Could you check a few things on this model? Use its own coordinates, in mm. Face numbers are marked on the shaded views. Give positions to 0.01 mm unless a question says otherwise; leave off trailing zeros. Loops run counter-clockwise (first coordinate to the right, second up) from the corner with the lowest first, then second, coordinate; pieces in that order, holes last. Notation, with made-up numbers: (71, 85.25) -> (124, 85.25) arc R18 cw to (124, 119.25) -> close; hole circle Ø5 at (-12, 87). An arc over 180 degrees is marked (long way). Write each question's results on one line, items separated by ' | '. Start each with the question number.
Q1. If we section it at A-A, the plane x = 0: List the corners of the cut face in (y, z) for me, plus the area to 3 significant figures.
Q2. Will these pins go through, and if not, where does the flat tip stop? P1, Ø1.5, axis at y = 3.5, z = -0.5, coming from the -X side; P2, Ø1.5, axis at x = -17, y = 3, coming from the +Z side; P3, Ø3, axis at x = 14.5, z = -14, coming from the +Y side.
Q3. If we section it at C-C, the plane y = 7: List the corners of the cut face in (x, z) for me.
Q4. If we section it at B-B, the plane z = 0: List the corners of the cut face in (x, y) for me.
Q5. We'd pull the mould along X, two halves only. Please class the marked faces 1, 2 and 3: released by +X, released by -X, zero draft, split by the parting line, or undercut.
Q6. If I drill on line 1 along X through (y, z) = (8.75, 0); line 2 along Y through (x, z) = (-15.5, 11.5); line 3 along Z through (x, y) = (-21.5, 9.5), over which ranges is the centre line in solid material (lowest first)?
from build123d import *

# Parameters (mm, degrees)
SKETCH1_R           = 32.5
BOSS_EXTRUDE4_DEPTH = 10
CUT_EXTRUDE1_REACH  = 12
SKETCH4_W           = 20
SKETCH4_H           = 5
SKETCH5_R           = 29
CUT_EXTRUDE3_DEPTH  = 2
FILLET1_R           = 1
FILLET2_R           = 1
CHAMFER1_SIZE       = 2


with BuildPart() as part:
    # Sketch1 → Boss-Extrude4 (new body)
    with BuildSketch(Plane(origin=(0, 0, 0), x_dir=(1, 0, 0), z_dir=(0, 1, 0))):
        with Locations(Location((0, 0, 0), (0, 0, 270))):  # turned: the seam where the file's is
            Circle(SKETCH1_R)
    extrude(amount=BOSS_EXTRUDE4_DEPTH)

    # Sketch4 → Cut-Extrude1 (cut, up to next)
    with BuildSketch(Plane(origin=(0, 10, 0), x_dir=(1, 0, 0), z_dir=(0, 1, 0)), mode=Mode.PRIVATE) as cut_extrude1_sk1:
        Rectangle(SKETCH4_W, SKETCH4_H)
    cut_extrude1_tool1 = extrude(cut_extrude1_sk1.sketch, amount=-CUT_EXTRUDE1_REACH, mode=Mode.PRIVATE) & part.part
    add(cut_extrude1_tool1.solids().sort_by_distance((0, 10, 0))[0], mode=Mode.SUBTRACT)

    # Sketch5 → Cut-Extrude3 (cut)
    with BuildSketch(Plane(origin=(0, 10, 0), x_dir=(1, 0, 0), z_dir=(0, 1, 0))):
        with Locations(Location((0, 0, 0), (0, 0, 270))):  # turned: the seam where the file's is
            Circle(SKETCH5_R)
    extrude(amount=-CUT_EXTRUDE3_DEPTH, mode=Mode.SUBTRACT)

    # Fillet1
    fillet1_edges = [part.edges().sort_by_distance(p)[0] for p in [
        (0, 10, -32.5),
    ]]
    fillet(fillet1_edges, radius=FILLET1_R)

    # Fillet2
    fillet2_edges = [part.edges().sort_by_distance(p)[0] for p in [
        (0, 10, -29),
    ]]
    fillet(fillet2_edges, radius=FILLET2_R)

    # Chamfer1
    chamfer1_edges = [part.edges().sort_by_distance(p)[0] for p in [
        (0, 0, -32.5),
    ]]
    chamfer(chamfer1_edges, length=CHAMFER1_SIZE)


solid = part.part
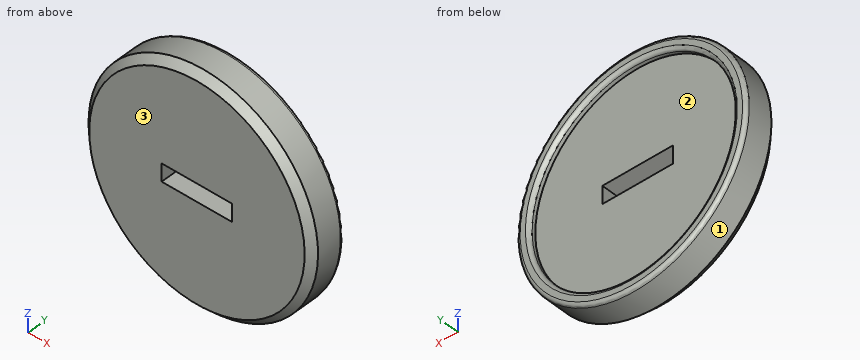
Final values:
1) outline: (0, -30.5) -> (2, -32.5) -> (9, -32.5) arc R1 ccw to (10, -31.5) -> (10, -30) arc R1 ccw to (9, -29) -> (8, -29) -> (8, -2.5) -> (0, -2.5) -> close; (0, 2.5) -> (8, 2.5) -> (8, 29) -> (9, 29) arc R1 ccw to (10, 30) -> (10, 31.5) arc R1 ccw to (9, 32.5) -> (2, 32.5) -> (0, 30.5) -> close | area: 489 mm²
2) P1: stops at x = -32.5 | P2: stops at z = 28.15 | P3: stops at y = 8
3) outline: circle Ø65 at (0, 0); hole (-10, -2.5) -> (10, -2.5) -> (10, 2.5) -> (-10, 2.5) -> close
4) outline: (-32.5, 2) -> (-30.5, 0) -> (-10, 0) -> (-10, 8) -> (-29, 8) -> (-29, 9) arc R1 ccw to (-30, 10) -> (-31.5, 10) arc R1 ccw to (-32.5, 9) -> close; (10, 0) -> (30.5, 0) -> (32.5, 2) -> (32.5, 9) arc R1 ccw to (31.5, 10) -> (30, 10) arc R1 ccw to (29, 9) -> (29, 8) -> (10, 8) -> close
5) face 1: split by the parting line | face 2: undercut | face 3: zero draft
6) line 1: x = -32.5 to -29, 29 to 32.5 | line 2: y = 0 to 8 | line 3: z = -24.19 to -19.66, 19.66 to 24.19
